Part model, mm, in its own coordinate system. Face numbers are marked on the shaded views. A direction names the side the tool comes from. Round coordinates to 2 decimals unless told otherwise and drop trailing zeros. Loops run counter-clockwise (first coordinate to the right, second up) from the corner with the lowest first, then second, coordinate; pieces in that order, holes last.
(1) Mould opens along Y. For the marked faces 1, 2 and 3 say: +Y half, -Y half, draft (parallel to the pull), parting line (faces both ways), or undercut.
(2) Cut at C-C on y = 13.5. List the corners of the cut face in (x, z), then the cut area to 3 significant figures.
(3) Cut at D-D on x = 7.5. List the corners of the cut face in (y, z).
(4) Cut at A-A on z = 1. List the corners of the cut face in (x, y), then the cut area to 3 significant figures.
(5) Flat gauge pins, fed straight in: pin 1 (1.6 mm diameter, centred on x = -10.5, y = 4.5, fed in from -Z); pin 2 (0.6 mm diameter, centred on x = 6, y = 4, fed in from -Z); pin 3 (3 mm diameter, centred on x = 1, y = 7.5, fed in from +Z). Where does each tip first touch, or does it go through?
(6) Tool access for the marked faces 4, 5 and 6: list every direction of +Z, -Z, +X, -X, +Y, -Y with a clear straight run to the whole face (end or side of a thin tool).
(7) Cut at B-B on x = -6.5. List the corners of the cut face in (y, z), then the cut area to 3 significant figures.
(8) Probe probe 1 along Y at (x, z) = (9, 4.25); probe 2 along X at (y, z) = (5.5, 3.5); probe 3 along X at (y, z) = (6, 9.25). List the from-to ranges inside material, lowest first.
from build123d import *

# Parameters (mm, degrees)
F1_DEPTH = 8
F3_R     = 2.5
F4_DEPTH = 2
F5_T     = -1.5


with BuildPart() as f1:
    # F0 (on Top) → F1 (new body)
    with BuildSketch(Plane.XY):
        Polygon((-14.1176469211, 8), (-14.1176469211, 0), (1.8823530789, 0), (8.3823530789, 0), (9.1710221022, 0), (17.8823530789, 0), (17.8823530789, 7.8231371145), (17.8823530789, 8.2882069845), (17.8823530789, 16), (-14.1176469211, 16), (-14.1176469211, 8.0556720495), align=None)
    extrude(amount=F1_DEPTH)

    # F3 (on offset) → F4 (join)
    with BuildSketch(Plane.XY.offset(8)):
        with Locations((-10.1726641878, 12.0353270322)):
            Circle(F3_R)
        with Locations((-10.1726641878, 4.043020308)):
            Circle(F3_R)
        with Locations((-2.180356998, 4.0956009179)):
            Circle(F3_R)
        with BuildLine():
            ThreePointArc((-2.180356998, 14.5879076421), (-3.948123951, 10.3201406892), (0.319643002, 12.0879076421))
            ThreePointArc((0.319643002, 12.0879076421), (-0.412590045, 13.8556745951), (-2.180356998, 14.5879076421))
        make_face()
        with Locations((5.8951441832, 12.0879076421)):
            Circle(F3_R)
        with Locations((5.8951441832, 4.0956009179)):
            Circle(F3_R)
        with Locations((13.887451373, 4.043020308)):
            Circle(F3_R)
        with Locations((13.887451373, 12.0353270322)):
            Circle(F3_R)
    extrude(amount=F4_DEPTH)

    # F5
    f5_openings = [f1.faces().sort_by_distance(p)[0] for p in [
        (1.882353, 8, 0),
    ]]
    offset(amount=F5_T, openings=f5_openings, kind=Kind.INTERSECTION)


solid = f1.part
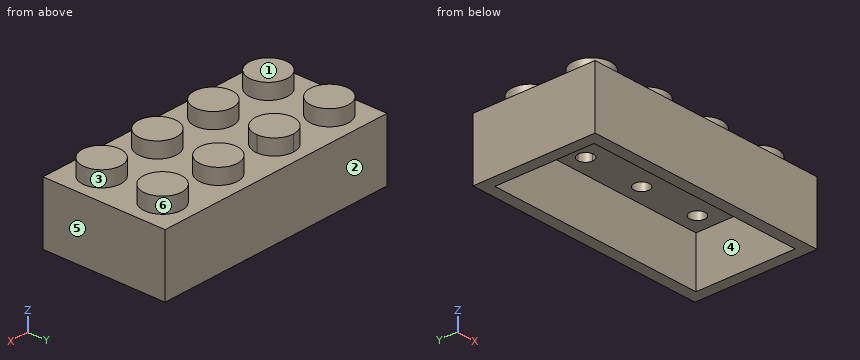
Final values:
1. face 1: draft
1. face 2: +Y half
1. face 3: undercut
2. outline: (-14.12, 0) - (-12.62, 0) - (-12.62, 6.5) - (16.38, 6.5) - (16.38, 0) - (17.88, 0) - (17.88, 8) - (15.91, 8) - (15.91, 10) - (11.86, 10) - (11.86, 8) - (7.96, 8) - (7.96, 10) - (3.83, 10) - (3.83, 8) - (-0.12, 8) - (-0.12, 10) - (-4.24, 10) - (-4.24, 8) - (-8.15, 8) - (-8.15, 10) - (-12.2, 10) - (-12.2, 8) - (-14.12, 8) - close
2. area: 100 mm2
3. outline: (0, 0) - (1.5, 0) - (1.5, 6.5) - (14.5, 6.5) - (14.5, 0) - (16, 0) - (16, 8) - (14, 8) - (14, 10) - (10.17, 10) - (10.17, 8) - (6.01, 8) - (6.01, 10) - (2.18, 10) - (2.18, 8) - (0, 8) - close
4. outline: (-14.12, 0) - (17.88, 0) - (17.88, 16) - (-14.12, 16) - close; hole (-12.62, 1.5) - (16.38, 1.5) - (16.38, 14.5) - (-12.62, 14.5) - close
4. area: 135 mm2
5. pin 1: stops at z = 6.5
5. pin 2: stops at z = 8.5
5. pin 3: stops at z = 8
6. face 4: -Z
6. face 5: +Z, -Z, +X, +Y, -Y
6. face 6: +Z
7. outline: (0, 0) - (1.5, 0) - (1.5, 6.5) - (14.5, 6.5) - (14.5, 0) - (16, 0) - (16, 8) - (0, 8) - close
7. area: 43.5 mm2
8. probe 1: y = 0 to 1.5, 14.5 to 16
8. probe 2: x = -14.12 to -12.62, 16.38 to 17.88
8. probe 3: x = -11.73 to -8.62, -3.8 to -0.56, 4.28 to 7.51, 12.33 to 15.44
